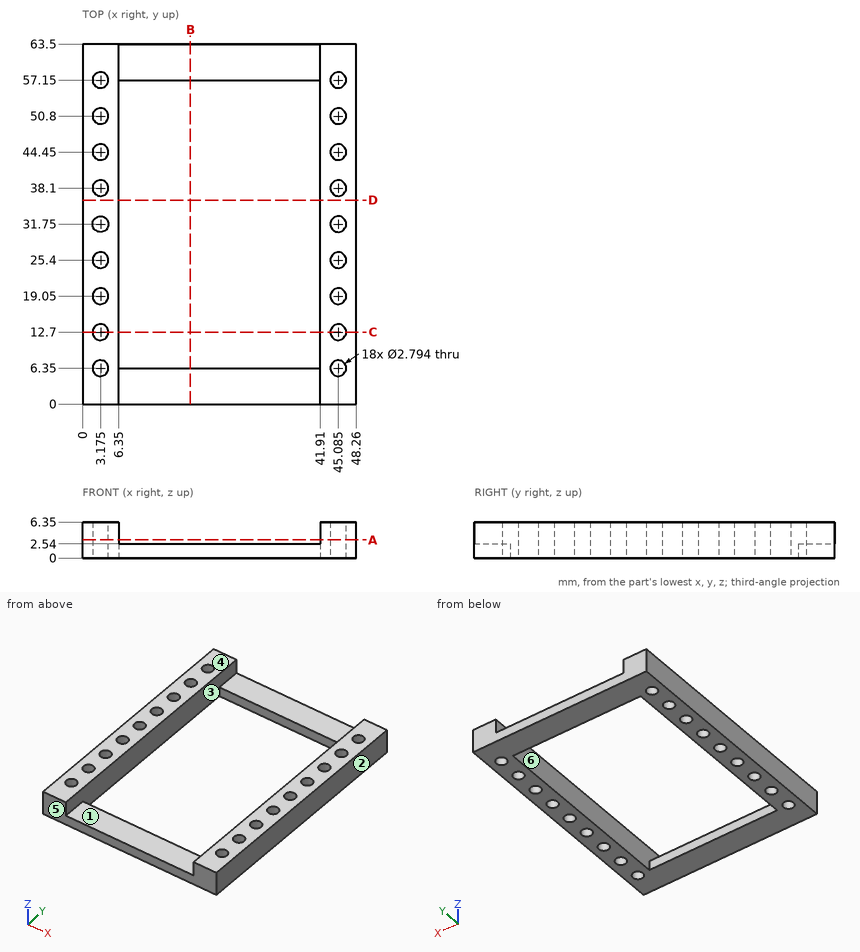
Verification items for this drawing (mm, ordinates from the low corner). A direction names the side the tool comes from. Coordinates: 2 decimals unless noted, no trailing zeros. Write each loop counter-clockwise with the first axis right and the second up, starting at its lowest first coordinate (ties: lowest second). Pieces come first, ordered by that corner, then holes. Notation, with made-up numbers: M -2,23.25 L 45,23.25 A21 ccw 45,38.25 Z; hole C -28.75,-12 d4. An arc over 180 degrees is marked long. Answer as a JSON object with one key per item and string values.
1. Tool access check on the marked faces 1, 2 and 3. Record the directions out of +Z, -Z, +X, -X, +Y, -Y that give a thin tool (end or side, any length) a straight path to the whole face; none if there is none.
Answers below:
{"face 1": "+Z, +Y, -Y", "face 2": "+Z, -Z, +X, +Y, -Y", "face 3": "+Z"}
2. Section check C-C, the plane y = 12.7. Enter the section's corners in (x, z).
Answers below:
{"outline": "M 0,0 L 1.78,0 L 1.78,6.35 L 0,6.35 Z; M 4.57,0 L 6.35,0 L 6.35,6.35 L 4.57,6.35 Z; M 41.91,0 L 43.69,0 L 43.69,6.35 L 41.91,6.35 Z; M 46.48,0 L 48.26,0 L 48.26,6.35 L 46.48,6.35 Z"}
3. Section check B-B, the plane x = 19. Enter the section's corners in (y, z), plus the area to 3 significant figures.
Answers below:
{"outline": "M 0,0 L 6.35,0 L 6.35,2.54 L 0,2.54 Z; M 57.15,0 L 63.5,0 L 63.5,2.54 L 57.15,2.54 Z", "area": "32.3 mm²"}
4. Section check D-D, the plane y = 36. Enter the section's corners in (x, z), plus the area to 3 significant figures.
Answers below:
{"outline": "M 0,0 L 6.35,0 L 6.35,6.35 L 0,6.35 Z; M 41.91,0 L 48.26,0 L 48.26,6.35 L 41.91,6.35 Z", "area": "80.6 mm²"}
5. Draft check along Y on the marked faces 4, 5 and 6. Enter one of: released by +Y, released by -Y, zero draft, split by the parting line, or undercut.
Answers below:
{"face 4": "zero draft", "face 5": "released by -Y", "face 6": "undercut"}
6. Go/stop test with a flat-tipped pin: pin 1 Ø10 at (x, y) = (14.5, 11) entering from +Z. Record where the tip stops, or that it passes through.
Answers below:
{"pin 1": "stops at z = 2.54"}
7. Section check A-A, the plane z = 3.25. Give the number of separate pieces and of enclosed holes in the cut face, plus the area to 3 significant figures.
Answers below:
{"separate pieces": "2", "enclosed holes": "18", "area": "696 mm²"}
8. Scan lines: L1, parallel to X at y = 38.1, z = 4; L2, parallel to Y at x = 28, z = 0.75; L3, parallel to X at y = 30, z = 3.25. Record each from-to range of solid material in increasing order.
Answers below:
{"L1": "x = 0 to 1.78, 4.57 to 6.35, 41.91 to 43.69, 46.48 to 48.26", "L2": "y = 0 to 6.35, 57.15 to 63.5", "L3": "x = 0 to 6.35, 41.91 to 48.26"}
